For this review, take the finished solid that the model builds, in its own axes (mm). A direction names the side the tool comes from. Round coordinates to 2 decimals unless told otherwise and drop trailing zeros. Write each loop counter-clockwise with the first axis right and the second up, starting at its lowest first coordinate (ties: lowest second). Pieces come first, ordered by that corner, then holes. Notation, with made-up numbers: (-21, 20.25) -> (23, 20.25) arc R17 cw to (23, 38.25) -> close; hole circle Ø6 at (40.5, 43). An arc over 180 degrees is marked (long way). Answer as CSV lines item,"result". Start each with the question number.
Item 1: Mouldability with a two-part tool opening along Y and no side actions: class faces 3 (the flat face through (0, -8.467, 4)), 4 (the flat face through (-7, 44.2, 27.94)), 5 (the flat face through (-7.23, 4.41, 3.79)), 6 (the cylindrical face through (43.61, 13.73, 13.77)) as +Y half, -Y half, draft (parallel to the pull), parting line (faces both ways), or undercut.
Item 2: Machinability: for faces 1 (the flat face through (-1, 1, 0)), 2 (the cylindrical face through (42.397, 13.352, 15.062)), which of the approach directions +Z, -Z, +X, -X, +Y, -Y give a long, thin tool a straight path to every point of the face, cutting with its end or side? Answer none if there is none.
Item 3: Take a section at A-A on y = -28. Give the boundary of the cut face in (x, z).
Item 4: For pin 1 Ø8 at (x, z) = (13, 7.5) entering from +Y; pin 2 Ø20.5 at (x, y) = (1, 8.5) entering from +Z; pin 3 Ø12 at (x, y) = (-22.5, -14) entering from -Z; pin 4 Ø2 at (x, y) = (20.5, -34) entering from +Z, all flat-tipped, find the tip position at first contact; note any pin that passes through.
Item 5: Take a section at B-B on z = 15.5. Give the boundary of the cut face in (x, y), then the cut area to 3 significant figures.
Item 6: Take a section at C-C on x = -4. Give the boundary of the cut face in (y, z), then the cut area to 3 significant figures.
Item 7: Wall thickness on probe 1 along Y at (x, z) = (0, 9.75); probe 2 along Z at (x, y) = (-20, -29); probe 3 along Z at (x, y) = (5, 5): over which ranges is each line inside the solid? List them lowest first. Write a range as from..to.
Item 8: Take a section at D-D on y = 0. Give the boundary of the cut face in (x, z), then the cut area to 3 significant figures.
```python
from build123d import *

# Parameters (mm, degrees)
F0_R     = 45.72
F0_R_2   = 44.45
F1_DEPTH = 27.94
F2_DEPTH = 2.54
F4_DEPTH = 2.54


with BuildPart() as f1:
    # F0 (on Top) → F1 (new body)
    with BuildSketch(Plane.XY):
        Circle(F0_R)
        Circle(F0_R_2, mode=Mode.SUBTRACT)
    extrude(amount=F1_DEPTH)

    # F0 (on Top) → F2 (join)
    with BuildSketch(Plane.XY):
        Circle(F0_R_2)
    extrude(amount=F2_DEPTH)

    # F3 (on face) → F4 (join)
    with BuildSketch(Plane.XY.offset(2.54)):
        Polygon((-14.664697, -8.466667), (14.664697, -8.466667), (0, 16.933333), align=None)
    extrude(amount=F4_DEPTH)


solid = f1.part
```
Output values:
1,face 3,"undercut"
1,face 4,"draft"
1,face 5,"undercut"
1,face 6,"parting line"
2,face 1,"-Z, +X, -X, +Y, -Y"
2,face 2,"+Z"
3,outline,"(-36.14, 0) -> (36.14, 0) -> (36.14, 27.94) -> (34.52, 27.94) -> (34.52, 2.54) -> (-34.52, 2.54) -> (-34.52, 27.94) -> (-36.14, 27.94) -> close"
4,pin 1,"stops at y = 44.83"
4,pin 2,"stops at z = 5.08"
4,pin 3,"stops at z = 0"
4,pin 4,"stops at z = 2.54"
5,outline,"circle Ø91.44 at (0, 0); hole circle Ø88.9 at (0, 0)"
5,area,"360 mm^2"
6,outline,"(-45.54, 0) -> (45.54, 0) -> (45.54, 27.94) -> (44.27, 27.94) -> (44.27, 2.54) -> (10.01, 2.54) -> (10.01, 5.08) -> (-8.47, 5.08) -> (-8.47, 2.54) -> (-44.27, 2.54) -> (-44.27, 27.94) -> (-45.54, 27.94) -> close"
6,area,"343 mm^2"
7,probe 1,"y = -45.72..-44.45, 44.45..45.72"
7,probe 2,"z = 0..2.54"
7,probe 3,"z = 0..5.08"
8,outline,"(-45.72, 0) -> (45.72, 0) -> (45.72, 27.94) -> (44.45, 27.94) -> (44.45, 2.54) -> (9.78, 2.54) -> (9.78, 5.08) -> (-9.78, 5.08) -> (-9.78, 2.54) -> (-44.45, 2.54) -> (-44.45, 27.94) -> (-45.72, 27.94) -> close"
8,area,"346 mm^2"
